from build123d import *

# Parameters (mm, degrees)
SKETCH_1_R          = 7.5
EXTRUDE_1_DEPTH     = 30
FILLET_1_R          = 0.75
SKETCH_2_R          = 2
CUT_EXTRUDE_1_DEPTH = 39.444765573
CHAMFER_1_SIZE      = 0.5


with BuildPart() as part:
    # 草图1 → 凸台-拉伸1 (new body)
    with BuildSketch(Plane.XY):
        Polygon((5, 11.25), (-5, 11.25), (-8.5, 5.75), (-15.5, 5.75), (-15.5, -4.25), (-17, -4.25), (-17, -11.25), (-7, -11.25), (-6, -9.75), (6, -9.75), (7, -11.25), (17, -11.25), (17, -4.25), (15.5, -4.25), (15.5, 5.75), (8.5, 5.75), align=None)
        with Locations((0, -0.75)):
            Circle(SKETCH_1_R, mode=Mode.SUBTRACT)
    extrude(amount=EXTRUDE_1_DEPTH)

    # 圆角1
    fillet_1_edges = [part.edges().sort_by_distance(p)[0] for p in [
        (-17, -11.25, 15),
        (-7, -11.25, 15),
        (-6, -9.75, 15),
        (7, -11.25, 15),
        (6, -9.75, 15),
        (17, -11.25, 15),
        (17, -4.25, 15),
        (15.5, -4.25, 15),
        (15.5, 5.75, 15),
        (5, 11.25, 15),
        (-5, 11.25, 15),
        (-17, -4.25, 15),
        (-15.5, -4.25, 15),
        (-15.5, 5.75, 15),
    ]]
    fillet(fillet_1_edges, radius=FILLET_1_R - 0.0001)  # a hair under: the kernel refuses the full size

    # 草图2 → 切除-拉伸1 (cut, through all)
    with BuildSketch(Plane(origin=(0, 5.75, 0), x_dir=(1, 0, 0), z_dir=(0, 1, 0))):
        with Locations(Location((-11.625, -6, 0), (0, 0, 180))):
            Circle(SKETCH_2_R)
        with Locations(Location((-11.625, -24, 0), (0, 0, 180))):
            Circle(SKETCH_2_R)
        with Locations((11.625, -24)):
            Circle(SKETCH_2_R)
        with Locations((11.625, -6)):
            Circle(SKETCH_2_R)
    extrude(amount=-CUT_EXTRUDE_1_DEPTH, mode=Mode.SUBTRACT)

    # 倒角1
    chamfer_1_edges = [part.edges().sort_by_distance(p)[0] for p in [
        (-9.625, -11.25, 24),
        (-9.625, 5.75, 24),
        (9.625, -11.25, 6),
        (9.625, 5.75, 6),
        (-9.625, -11.25, 6),
        (-9.625, 5.75, 6),
        (9.625, -11.25, 24),
        (9.625, 5.75, 24),
    ]]
    chamfer(chamfer_1_edges, length=CHAMFER_1_SIZE)


solid = part.part
Source: CAD feature listing. Evaluate the final solid. Frame: model axes, mm. A direction names the side the tool comes from. Round coordinates to 2 decimals unless told otherwise and drop trailing zeros. Write each loop counter-clockwise with the first axis right and the second up, starting at its lowest first coordinate (ties: lowest second). Pieces come first, ordered by that corner, then holes. Notation, with made-up numbers: M -18.75,-4 L 30.25,-4 A25 ccw 30.25,28 Z; hole C 68.5,-8 d1. An arc over 180 degrees is marked long. One line per item, written item: value. Start each with the question number.
Item 1: Section query B-B (y = -0.75). Return the cut outline in (x, z) (3 decimals), plus the area to 3 significant figures.
Item 2: Set-up query: faces 1 (the flat face through (6.5, -10.5, 14.8)), 2 (the flat face through (12, 5.75, 15)), 3 (the flat face through (-12, 5.75, 15)). Return all of +Z, -Z, +X, -X, +Y, -Y with unobstructed straight access to the full face (end or side cutting, diameter ignored); none if empty.
Item 3: Mould query, pull axis X, two halves, no side actions, for faces 4 (the flat face through (-6.84, 8.36, 14.79)), 5 (the cylindrical face through (-9.627, -2.638, 6.088)), 6 (the flat face through (12, -11.25, 15)). Classes: pulls with the +X half, pulls with the -X half, needs draft (parallel to the pull), parting line crosses it, or undercut.
Item 4: Ray query, L1, parallel to Z at x = -11, y = -8.25; L2, parallel to Y at x = 0, z = 6.25; L3, parallel to Z at x = 13, y = -3.25. Return the intervals inside material, ascending. Write a range as from..to.
Item 5: Section query A-A (x = 0). Return the cut outline in (y, z), plus the area to 3 significant figures.
Item 6: Section query D-D (y = -5.5). Return the cut outline in (x, z) (3 decimals).
Item 7: Pin query (flat end, axial travel): pin 1 (4.5 mm diameter, centred on y = 1.5, z = 13.5, fed in from -X); pin 2 (6.5 mm diameter, centred on x = -11.625, z = 6, fed in from +Y); pin 3 (3 mm diameter, centred on x = -11.625, z = 24, fed in from -Y); pin 4 (4.5 mm diameter, centred on x = 11.625, z = 24, fed in from +Y). Return the tip coordinate at first contact, or that it passes through.
Result set:
1. outline: M -15.5,0 L -7.5,0 L -7.5,30 L -15.5,30 Z; M 7.5,0 L 15.5,0 L 15.5,30 L 7.5,30 Z; hole C -11.625,6 d4; hole C -11.625,24 d4; hole C 11.625,6 d4; hole C 11.625,24 d4
1. area: 430 mm²
2. face 1: +Z, -Z, -Y
2. face 2: +Z, -Z, +X, +Y
2. face 3: +Z, -Z, -X, +Y
3. face 4: pulls with the -X half
3. face 5: undercut
3. face 6: needs draft
4. L1: z = 0..4.1, 7.9..22.1, 25.9..30
4. L2: y = -9.75..-8.25, 6.75..11.25
4. L3: z = 0..4.55, 7.45..22.55, 25.45..30
5. outline: M -9.75,0 L -8.25,0 L -8.25,30 L -9.75,30 Z; M 6.75,0 L 11.25,0 L 11.25,30 L 6.75,30 Z
5. area: 180 mm²
6. outline: M -17,0 L -5.804,0 L -5.804,30 L -17,30 Z; M 5.804,0 L 17,0 L 17,30 L 5.804,30 Z; hole C -11.625,6 d4; hole C -11.625,24 d4; hole C 11.625,6 d4; hole C 11.625,24 d4
7. pin 1: stops at x = -15.5
7. pin 2: stops at y = 5.95
7. pin 3: passes through
7. pin 4: stops at y = 5.5
